Read the model definition and answer for the solid it produces. Units are mm, in the model's axes. Face numbers are marked on the shaded views. A direction names the side the tool comes from. Coordinates: 2 decimals unless noted, no trailing zeros. Loops run counter-clockwise (first coordinate to the right, second up) from the corner with the lowest first, then second, coordinate; pieces in that order, holes last.
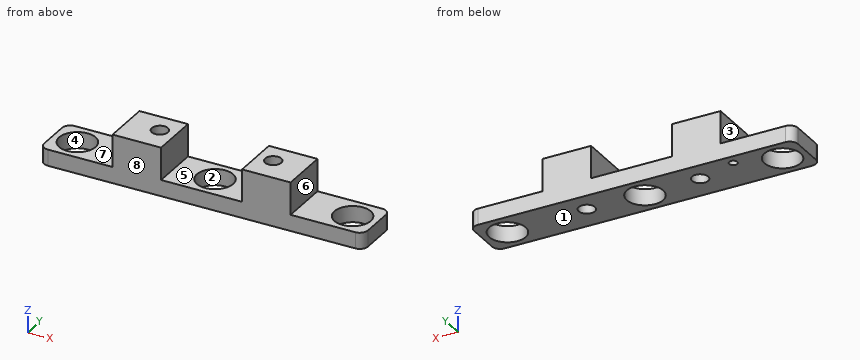
Autodesk Inventor part; units mm, degrees
ref_plane "YZ Plane" through (0, 0, 0) normal (1, 0, 0) x (0, 1, 0)
ref_plane "XZ Plane" through (0, 0, 0) normal (0, 1, 0) x (-1, 0, 0)
ref_plane "XY Plane" through (0, 0, 0) normal (0, 0, 1) x (1, 0, 0)
sketch "Sketch1" plane through (0, 0, 0) normal (0, 0, 1) x (1, 0, 0)
  line L0 (-20, -3) -> (20, -3) construction
  circle A0 centre (-17, 0) radius 2.25
  circle A1 centre (17, 0) radius 2.25
  circle A2 centre (0, 0) radius 2.25
  circle A3 centre (-7, 0.3446) radius 1
  circle A4 centre (7, 0.3446) radius 1
  line L1 (-23.9554, 0) -> (25.6733, 0) construction
  line L2 (0, 11.421) -> (0, -11.2937) construction
  line L3 (-20, -3) -> (20, -3)
  line L4 (20, -3) -> (20, 3)
  line L5 (20, 3) -> (-20, 3)
  line L6 (-20, 3) -> (-20, -3)
  circle A5 centre (-11.8345, 1.6861) radius 0.5
  line L7 (-11, 3) -> (-5, 3)
  line L8 (-5, 3) -> (-5, -3)
  line L9 (-5, -3) -> (-11, -3)
  line L10 (-11, -3) -> (-11, 3)
  line L11 (5, 3) -> (11, 3)
  line L12 (11, 3) -> (11, -3)
  line L13 (11, -3) -> (5, -3)
  line L14 (5, -3) -> (5, 3)
  point P0 (0, 0)
  point P1 (0, -3)
  point P2 (0, -3)
  point P3 (-2.8751, -5.808)
  point P4 (2.8751, -5.808)
  dimension "d0" = 40
  dimension "d1" = 4.5
  dimension "d2" = 4.5
  dimension "d3" = 3
  dimension "d4" = 4.5
  dimension "d5" = 3
  dimension "d6" = 3.3446
  dimension "d7" = 3.3446
  dimension "d8" = 3
  dimension "d9" = 17
  dimension "d10" = 17
  dimension "d11" = 3
  dimension "d12" = 3
  dimension "d13" = 3
  dimension "d14" = 3
  dimension "d16" = 1
  dimension "d20" = 6
  dimension "d22" = 5
  dimension "d23" = 5
  dimension "d24" = 6
extrude "Extrusion1" add sketch "Sketch1" along normal blind 2
fillet "Fillet1" radius 1 4 edges at (-20, 3, 1) (-20, -3, 1) (20, 3, 1) (20, -3, 1)
extrude "Extrusion2" add sketch "Sketch1" along normal blind 6 contours L10 L5 L8 L3 | L14 L5 L12 L3
properties part number "Bar_Extruded"
Q1. Which of the six approach directions +Z, -Z, +X, -X, +Y, -Y give full straight-line access (tool end or side, diameter ignored) to the marked faces 4, 5, 6, 7 and 8?
Findings below:
face 4: +Z, -Z
face 5: +Z, +Y, -Y
face 6: +Z, +X, +Y, -Y
face 7: +Z, -X, +Y, -Y
face 8: +Z, -Z, +X, -X, -Y
Q2. Flat-ended cylindrical pins translate along their axes: pin 1 Ø1.2 at (y, z) = (0.5, 4) entering from +X; pin 2 Ø3 at (y, z) = (1, 4) entering from -X; pin 3 Ø2.5 at (x, y) = (7, 0.34) entering from +Z; pin 4 Ø1.8 at (x, y) = (-17.5, -1) entering from +Z (1 decimal). Find the tip coordinate at first contact, or state that the pin passes through.
Findings below:
pin 1: stops at x = 11
pin 2: stops at x = -11
pin 3: stops at z = 6
pin 4: passes through
Q3. A cutting plane is placed at B-B (y = 2.6). Give the vertices of the cut face in (x, z).
Findings below:
outline: (-19.8, 0) - (19.8, 0) - (19.8, 2) - (11, 2) - (11, 6) - (5, 6) - (5, 2) - (-5, 2) - (-5, 6) - (-11, 6) - (-11, 2) - (-19.8, 2) - close
Q4. A cutting plane is placed at D-D (y = 0). Count the separate pieces of the cut face and the enclosed holes in it, then the cut area to 3 significant figures.
Findings below:
separate pieces: 6
enclosed holes: 0
area: 78.5 mm2
Q5. Straight lines are drawn through the part: probe 1 along X at (y, z) = (2.45, 2.7); probe 2 along X at (y, z) = (0.2, 4.7); probe 3 along Y at (x, z) = (0, 0.6). For each, find the intervals that lie inside material, in ascending order.
Findings below:
probe 1: x = -11 to -5, 5 to 11
probe 2: x = -11 to -7.99, -6.01 to -5, 5 to 6.01, 7.99 to 11
probe 3: y = -3 to -2.25, 2.25 to 3
Q6. A cutting plane is placed at A-A (x = 0). Give the vertices of the cut face in (y, z).
Findings below:
outline: (-3, 0) - (-2.25, 0) - (-2.25, 2) - (-3, 2) - close; (2.25, 0) - (3, 0) - (3, 2) - (2.25, 2) - close
Q7. A cutting plane is placed at C-C (z = 5.65). Give the vertices of the cut face in (x, y), then the cut area to 3 significant figures.
Findings below:
outline: (-11, -3) - (-5, -3) - (-5, 3) - (-11, 3) - close; (5, -3) - (11, -3) - (11, 3) - (5, 3) - close; hole circle Ø2 at (-7, 0.34); hole circle Ø2 at (7, 0.34)
area: 65.7 mm2
Q8. Determine the mould class of the marked faces 1, 2 and 3 for opening direction X: +X half, -X half, draft (parallel to the pull), parting line (faces both ways), or undercut.
Findings below:
face 1: draft
face 2: undercut
face 3: -X half
